Check sheet for the modelled part. Datum: model origin and axes. Units: mm. A direction names the side the tool comes from. Round coordinates to 2 decimals unless told otherwise and drop trailing zeros. Loops run counter-clockwise (first coordinate to the right, second up) from the corner with the lowest first, then second, coordinate; pieces in that order, holes last. Notation, with made-up numbers: (5, 62.5) -> (48, 62.5) arc R24 cw to (48, 72.5) -> close; hole circle Ø10 at (-29, -9.75). An arc over 180 degrees is marked (long way). Return JSON: item names as keys, results as strings.
from build123d import *

# Parameters (mm, degrees)
F1_DEPTH = 10
F2_R     = 1.3
F3_DEPTH = 2


# Not quite as in the source:
# - a feature names something its author has since deleted; it is built from what else it names


with BuildPart() as f1:
    # F0 (on Top) → F1 (new body)
    with BuildSketch(Plane.XY):
        Polygon((-5, -6.5), (5, -6.5), (5, 6.5), (-5, 6.5), (-5, 4.5), (-3, 4.5), (3, 4.5), (3, -4.5), (-3, -4.5), (-5, -4.5), align=None)
    extrude(amount=F1_DEPTH)

    # F2 (on face) → F3 (cut, through all)
    with BuildSketch(Plane.XZ.offset(6.5)):
        with Locations((-1, 5)):
            Circle(F2_R)
    extrude(amount=-F3_DEPTH, mode=Mode.SUBTRACT)


solid = f1.part
Q1. Section check D-D (y = -5.25). Record the boundary of the cut face in (x, z), then the cut area to 3 significant figures.
Results list:
{"outline": "(-5, 0) -> (5, 0) -> (5, 10) -> (-5, 10) -> close; hole circle Ø2.6 at (-1, 5)", "area": "94.7 mm^2"}
Q2. Tool access check on faces 1 (the flat face through (5, 0, 5)), 2 (the cylindrical face through (-1.28, -5.51, 3.73)), 3 (the flat face through (3, 0, 5)). Record the directions out of +Z, -Z, +X, -X, +Y, -Y that give a thin tool (end or side, any length) a straight path to the whole face; none if there is none.
Results list:
{"face 1": "+Z, -Z, +X, +Y, -Y", "face 2": "-Y", "face 3": "+Z, -Z, -X"}
Q3. Section check A-A (x = -2.5). Record the boundary of the cut face in (y, z), then the cut area to 3 significant figures.
Results list:
{"outline": "(-6.5, 0) -> (-4.5, 0) -> (-4.5, 10) -> (-6.5, 10) -> close; (4.5, 0) -> (6.5, 0) -> (6.5, 10) -> (4.5, 10) -> close", "area": "40.0 mm^2"}
Q4. Material ranges on line 1 (Y direction, x = -2.5, z = 4); line 2 (Z direction, x = -1, y = -5.5); line 3 (X direction, y = -3.5, z = 9.25), recorded low to high.
Results list:
{"line 1": "-6.5 to -4.5, 4.5 to 6.5", "line 2": "0 to 3.7, 6.3 to 10", "line 3": "3 to 5"}
Q5. Go/stop test with flat-tipped pins: pin 1 (1 mm diameter, centred on x = 1, y = -1.5, fed in from +Z); pin 2 (4 mm diameter, centred on y = 0.5, z = 5, fed in from -X). Record where each tip stops, or that it passes through.
Results list:
{"pin 1": "through", "pin 2": "x = 3"}
Q6. Draft check along Y on faces 4 (the flat face through (3.3, 0.1, 10)), 5 (the flat face through (-0.1, -4.5, 3.8)), 6 (the flat face through (0, 6.5, 5)). Enter one of: released by +Y, released by -Y, zero draft, split by the parting line, or undercut.
Results list:
{"face 4": "zero draft", "face 5": "undercut", "face 6": "released by +Y"}
Q7. Section check C-C (z = 4.75). Record the boundary of the cut face in (x, y).
Results list:
{"outline": "(-5, -6.5) -> (-2.28, -6.5) -> (-2.28, -4.5) -> (-5, -4.5) -> close; (-5, 4.5) -> (3, 4.5) -> (3, -4.5) -> (0.28, -4.5) -> (0.28, -6.5) -> (5, -6.5) -> (5, 6.5) -> (-5, 6.5) -> close"}
Q8. Section check B-B (x = -1). Record the boundary of the cut face in (y, z).
Results list:
{"outline": "(-6.5, 0) -> (-4.5, 0) -> (-4.5, 3.7) -> (-6.5, 3.7) -> close; (-6.5, 6.3) -> (-4.5, 6.3) -> (-4.5, 10) -> (-6.5, 10) -> close; (4.5, 0) -> (6.5, 0) -> (6.5, 10) -> (4.5, 10) -> close"}
